Geometry check sheet. Reference: the model listing, model coordinates, mm. Give positions to 0.01 mm unless a question says otherwise; leave off trailing zeros. Write each loop counter-clockwise with the first axis right and the second up, starting at its lowest first coordinate (ties: lowest second). Pieces come first, ordered by that corner, then holes. Notation, with made-up numbers: M 28,54.25 L 62,54.25 A21 cw 62,76.25 Z; hole C 32,-24 d6. An arc over 180 degrees is marked long. One line per item, written item: value. Start each with the question number.
1. Gauge pin test, flat ends, axial feed: pin 1 (4 mm diameter, centred on x = 105, y = 29.05, fed in from -Z); pin 2 (5 mm diameter, centred on x = 71, z = 5.5, fed in from +Y); pin 3 (1.5 mm diameter, centred on y = -121.5, z = 4, fed in from +X); pin 4 (3 mm diameter, centred on y = -26.5, z = 7, fed in from -X). Record the tip position at first contact, or that the pin passes through.
2. Cross-section at A-A on y = 0. Record the cut outline in (x, z), then the cut area to 3 significant figures.
3. Scan lines: line 1 (Y direction, x = 157.5, z = 2.5); line 2 (Y direction, x = 105, z = 5.25); line 3 (X direction, y = -3, z = 8.5). Record each from-to range of solid material in increasing order.
4. Cross-section at B-B on z = 4. Count the separate pieces of the cut face and the enclosed holes in it, then the cut area to 3 significant figures.
from build123d import *

# Parameters (mm, degrees)
ESQUISSE1_R             = 47.5
BOSS_EXTRU_1_DEPTH      = 10
ESQUISSE3_W             = 100
ESQUISSE3_H             = 10
ENL_V_MAT_EXTRU_1_DEPTH = 11
ESQUISSE4_R             = 2.5
ENL_V_MAT_EXTRU_2_DEPTH = 11
ESQUISSE6_W             = 150
ESQUISSE6_H             = 120
BOSS_EXTRU_2_DEPTH      = 10
ESQUISSE7_W             = 10
ESQUISSE7_H             = 50
ESQUISSE7_W_2           = 50
ESQUISSE7_H_2           = 9.570800355
ENL_V_MAT_EXTRU_3_DEPTH = 10
ENL_V_MAT_EXTRU_4_DEPTH = 10
ESQUISSE9_W             = 10
ESQUISSE9_H             = 50
BOSS_EXTRU_3_DEPTH      = 10


with BuildPart() as part:
    # Esquisse1 → Boss.-Extru.1 (new body)
    with BuildSketch(Plane.XY):
        Polygon((-310, -75.642859016), (0, 414.561180135), (310, -75.642859016), align=None)
        with Locations((-157.5, 0)):
            Circle(ESQUISSE1_R, mode=Mode.SUBTRACT)
        with Locations((-52.5, 0)):
            Circle(ESQUISSE1_R, mode=Mode.SUBTRACT)
        with Locations((52.5, 0)):
            Circle(ESQUISSE1_R, mode=Mode.SUBTRACT)
        with Locations((157.5, 0)):
            Circle(ESQUISSE1_R, mode=Mode.SUBTRACT)
        with Locations((-105, 90.932667397)):
            Circle(ESQUISSE1_R, mode=Mode.SUBTRACT)
        with Locations((0, 90.932667397)):
            Circle(ESQUISSE1_R, mode=Mode.SUBTRACT)
        with Locations((105, 90.932667397)):
            Circle(ESQUISSE1_R, mode=Mode.SUBTRACT)
        with Locations((-52.5, 181.865334795)):
            Circle(ESQUISSE1_R, mode=Mode.SUBTRACT)
        with Locations((52.5, 181.865334795)):
            Circle(ESQUISSE1_R, mode=Mode.SUBTRACT)
        with Locations((0, 272.798002192)):
            Circle(ESQUISSE1_R, mode=Mode.SUBTRACT)
    extrude(amount=BOSS_EXTRU_1_DEPTH)

    # Esquisse3 → Enlèv. mat.-Extru.1 (cut, through all)
    with BuildSketch(Plane.XY.offset(10)):
        Polygon((-269.913793103, -12.254405678), (-261.461999325, -17.599233264), (-208.013723463, 66.918704521), (-216.465517241, 72.263532107), align=None)
        Polygon((-181.724137931, 127.200191667), (-173.272344153, 121.855364081), (-119.82406829, 206.373301865), (-128.275862069, 211.718129452), align=None)
        Polygon((-93.534482759, 266.654789012), (-85.08268898, 261.309961425), (-31.634413118, 345.82789921), (-40.086206897, 351.172726796), align=None)
        Polygon((269.913793103, -12.254405678), (261.461999325, -17.599233264), (208.013723463, 66.918704521), (216.465517241, 72.263532107), align=None)
        Polygon((181.724137931, 127.200191667), (173.272344153, 121.855364081), (119.82406829, 206.373301865), (128.275862069, 211.718129452), align=None)
        Polygon((93.534482759, 266.654789012), (85.08268898, 261.309961425), (31.634413118, 345.82789921), (40.086206897, 351.172726796), align=None)
        with Locations((-160, -70.642859016)):
            Rectangle(ESQUISSE3_W, ESQUISSE3_H)
        with Locations((160, -70.642859016)):
            Rectangle(ESQUISSE3_W, ESQUISSE3_H)
    extrude(amount=-ENL_V_MAT_EXTRU_1_DEPTH, mode=Mode.SUBTRACT)

    # Esquisse4 → Enlèv. mat.-Extru.2 (cut, through all)
    with BuildSketch(Plane.XY.offset(10)):
        with Locations((-157.5, -55.642859016)):
            Circle(ESQUISSE4_R)
        with Locations((-52.5, -55.642859016)):
            Circle(ESQUISSE4_R)
        with Locations((52.5, -55.642859016)):
            Circle(ESQUISSE4_R)
        with Locations((157.5, -55.642859016)):
            Circle(ESQUISSE4_R)
        with Locations((-105, 29.047375097)):
            Circle(ESQUISSE4_R)
        with Locations((0, 29.047375097)):
            Circle(ESQUISSE4_R)
        with Locations((105, 29.047375097)):
            Circle(ESQUISSE4_R)
        with Locations((-52.5, 119.980042494)):
            Circle(ESQUISSE4_R)
        with Locations((52.5, 119.980042494)):
            Circle(ESQUISSE4_R)
        with Locations((0, 210.912709891)):
            Circle(ESQUISSE4_R)
    extrude(amount=-ENL_V_MAT_EXTRU_2_DEPTH, mode=Mode.SUBTRACT)

    # Esquisse6 → Boss.-Extru.2 (add)
    with BuildSketch(Plane.XY.offset(10)):
        with Locations((0, -135.642859016)):
            Rectangle(ESQUISSE6_W, ESQUISSE6_H)
    extrude(amount=-BOSS_EXTRU_2_DEPTH)

    # Esquisse7 → Enlèv. mat.-Extru.3 (cut)
    with BuildSketch(Plane.XY.offset(10)):
        with Locations((-70, -135.642859016)):
            Rectangle(ESQUISSE7_W, ESQUISSE7_H)
        with Locations((0, -190.857458839)):
            Rectangle(ESQUISSE7_W_2, ESQUISSE7_H_2)
        with Locations((70, -135.642859016)):
            Rectangle(ESQUISSE7_W, ESQUISSE7_H)
    extrude(amount=-ENL_V_MAT_EXTRU_3_DEPTH, mode=Mode.SUBTRACT)

    # Esquisse8 → Enlèv. mat.-Extru.4 (cut)
    with BuildSketch(Plane.XY.offset(10)):
        Polygon((0, -217.346828515), (0, 109.461180135), (292.569272736, 109.461180135), (292.569272736, 414.561180135), (0, 414.561180135), (-356.657737224, 414.561180135), (-356.657737224, -217.346828515), align=None)
    extrude(amount=-ENL_V_MAT_EXTRU_4_DEPTH, mode=Mode.SUBTRACT)

    # Esquisse9 → Boss.-Extru.3 (add)
    with BuildSketch(Plane.XY.offset(10)):
        with Locations((-5, -111.072058661)):
            Rectangle(ESQUISSE9_W, ESQUISSE9_H)
    extrude(amount=-BOSS_EXTRU_3_DEPTH)


solid = part.part
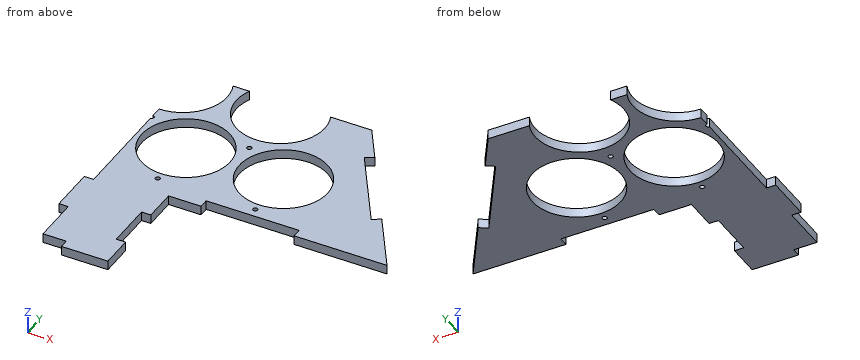
Report:
1. pin 1: passes through
1. pin 2: stops at y = 60.54
1. pin 3: stops at x = 65
1. pin 4: stops at x = 0
2. outline: M 0,0 L 5,0 L 5,10 L 0,10 Z; M 100,0 L 110,0 L 110,10 L 100,10 Z; M 205,0 L 250.33,0 L 250.33,10 L 205,10 Z
2. area: 603 mm^2
3. line 1: y = -65.64 to -58.14, -53.14 to -47.5, 47.5 to 109.46
3. line 2: y = -75.64 to 26.55, 31.55 to 43.43
3. line 3: x = 0 to 5.09, 99.91 to 110.09, 204.91 to 252.23
4. separate pieces: 1
4. enclosed holes: 5
4. area: 31,200 mm^2
